Design review of the part built by this model. Coordinates are the model's own, in mm. Face numbers are marked on the shaded views. A direction names the side the tool comes from. Give positions to 0.01 mm unless a question says otherwise; leave off trailing zeros. Write each loop counter-clockwise with the first axis right and the second up, starting at its lowest first coordinate (ties: lowest second). Pieces come first, ordered by that corner, then holes. Notation, with made-up numbers: (-8, 77.25) -> (2, 77.25) arc R32 cw to (2, 106.25) -> close; hole circle Ø4 at (-9.5, 33.25). An arc over 180 degrees is marked (long way). Return JSON: item names as keys, results as strings. Group by question number.
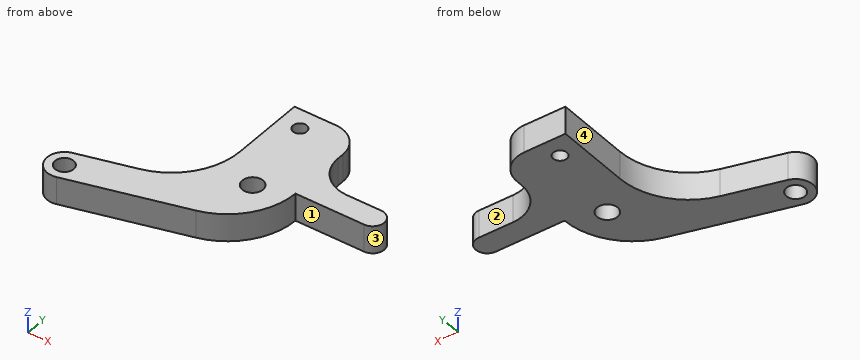
from build123d import *

# Parameters (mm, degrees)
SKETCH1_R           = 1.5
SKETCH1_R_2         = 1
SKETCH1_R_3         = 1.35
BOSS_EXTRUDE1_DEPTH = 4
FILLET1_R           = 10
FILLET2_R           = 10
FILLET3_R           = 5
FILLET4_R           = 4


with BuildPart() as part:
    # Sketch1 → Boss-Extrude1 (new body)
    with BuildSketch(Plane.XY):
        with BuildLine():
            Line((15, 5), (5, 5))
            Line((5, 5), (5, 15))
            Line((5, 15), (-5, 15))
            Line((-5, 15), (-5, -3.392571663))
            Line((-5, -3.392571663), (-20.647047613, -7.585185434))
            ThreePointArc((-20.647047613, -7.585185434), (-22.414814566, -10.647047613), (-19.352952387, -12.414814566))
            Line((-19.352952387, -12.414814566), (5, -5.88946064))
            Line((5, -5.88946064), (5, 1.658780206))
            Line((5, 1.658780206), (15, 1.658780206))
            ThreePointArc((15, 1.658780206), (16.670609897, 3.329390103), (15, 5))
        make_face()
        Circle(SKETCH1_R, mode=Mode.SUBTRACT)
        with Locations((-2, 12)):
            Circle(SKETCH1_R_2, mode=Mode.SUBTRACT)
        with Locations((-20, -10)):
            Circle(SKETCH1_R_3, mode=Mode.SUBTRACT)
    extrude(amount=BOSS_EXTRUDE1_DEPTH)

    # Fillet1
    # the kernel refuses this fillet: 10 mm, written as the material it takes off along each edge
    with BuildSketch(Plane(origin=(5, -5.88946064, -19.183174699), x_dir=(-0.965925826289069, -0.2588190451025183, 0), z_dir=(0, 0, 1))) as fillet1_piece_1_section:
        with BuildLine():
            CenterArc((FILLET1_R * 0.767326987979, -FILLET1_R), FILLET1_R, 90, 75)
            Line((-FILLET1_R * 0.19859883831, -FILLET1_R * 0.741180954897), (0, 0))
            Line((0, 0), (FILLET1_R * 0.767326987979, 0))
        make_face()
    fillet1_piece_1 = extrude(amount=42.366349399, mode=Mode.PRIVATE)
    fillet1_piece_1 = split(fillet1_piece_1, bisect_by=Plane(origin=(3.36090957, 1.658780206, 2), z_dir=(0, -1, 0)), keep=Keep.TOP, mode=Mode.PRIVATE)
    add(fillet1_piece_1, mode=Mode.SUBTRACT)

    # Fillet2
    fillet2_edges = [part.edges().sort_by_distance(p)[0] for p in [
        (-5, -3.392571663, 2),
    ]]
    fillet(fillet2_edges, radius=FILLET2_R)

    # Fillet3
    fillet3_edges = [part.edges().sort_by_distance(p)[0] for p in [
        (5, 5, 2),
    ]]
    fillet(fillet3_edges, radius=FILLET3_R)

    # Fillet4
    fillet4_edges = [part.edges().sort_by_distance(p)[0] for p in [
        (5, 15, 2),
    ]]
    fillet(fillet4_edges, radius=FILLET4_R)


solid = part.part
Q1. For L1, parallel to Y at x = 11.5, z = 2.95; L2, parallel to Y at x = -2, z = 2; L3, parallel to Y at x = -20, z = 1.25, list the stretches that pass through material, from the lowest coordinate up. Write a range as from..to.
Q2. Take a section at B-B, the plane x = 0. Give the boundary of the cut face in (y, z), plus the area to 3 significant figures.
Q3. Take a section at D-D, the plane x = 6. Give the boundary of the cut face in (y, z).
Q4. Take a section at A-A, the plane z = 1.4. Give the boundary of the cut face in (x, y), plus the area to 3 significant figures.
Q5. Tool access review of the marked faces 1, 2, 3 and 4: name each direction out of +Z, -Z, +X, -X, +Y, -Y from which nothing blocks a thin tool from reaching the whole face with its end or side.
Q6. Take a section at C-C, the plane y = 0. Give the boundary of the cut face in (x, z), plus the area to 3 significant figures.
Q7. Insertion check: pin 1 (2 mm diameter, centred on y = 11, z = 1.5, fed in from -X); pin 2 (0.5 mm diameter, centred on y = 10.5, z = 2.5, fed in from +X); pin 3 (1.2 mm diameter, centred on x = 13.5, z = 1, fed in from +Y). Each pin has a flat end and moves straight along its axis. Give the tip position at first contact, or say it passes through.
Final values:
{
 "1": {"L1": "y = 1.66..5", "L2": "y = -7.76..11, 13..15", "L3": "y = -12.5..-11.35, -8.65..-7.41"},
 "2": {"outline": "(-6.88, 0) -> (-1.5, 0) -> (-1.5, 4) -> (-6.88, 4) -> close; (1.5, 0) -> (15, 0) -> (15, 4) -> (1.5, 4) -> close", "area": "75.5 mm²"},
 "3": {"outline": "(1.66, 0) -> (7, 0) -> (7, 4) -> (1.66, 4) -> close"},
 "4": {"outline": "(-20.65, -7.59) arc R2.5 ccw to (-19.35, -12.41) -> (-2.41, -7.88) arc R10 ccw to (5, 1.66) -> (15, 1.66) arc R1.67 ccw to (15, 5) -> (10, 5) arc R5 cw to (5, 10) -> (5, 11) arc R4 ccw to (1, 15) -> (-5, 15) -> (-5, 4.28) arc R10 cw to (-12.41, -5.38) -> close; hole circle Ø2.7 at (-20, -10); hole circle Ø2 at (-2, 12); hole circle Ø3 at (0, 0)", "area": "334 mm²"},
 "5": {"face 1": "+Z, -Z, +X, -Y", "face 2": "+Z, -Z, +X, +Y", "face 3": "+Z, -Z, +X", "face 4": "+Z, -Z, -X, +Y"},
 "6": {"outline": "(-5.96, 0) -> (-1.5, 0) -> (-1.5, 4) -> (-5.96, 4) -> close; (1.5, 0) -> (4.84, 0) -> (4.84, 4) -> (1.5, 4) -> close", "area": "31.2 mm²"},
 "7": {"pin 1": "stops at x = -5", "pin 2": "stops at x = 5", "pin 3": "stops at y = 5"}
}
